```python
from build123d import *

# Parameters (mm, degrees)
SKETCH1_W           = 60
SKETCH1_H           = 400
BOSS_EXTRUDE1_DEPTH = 3
SKETCH2_W           = 3
SKETCH2_H           = 40
SKETCH2_W_2         = 10
SKETCH2_H_2         = 3
SKETCH2_W_3         = 7
SKETCH2_W_4         = 20
CUT_EXTRUDE3_DEPTH  = 3
SKETCH3_W           = 3
SKETCH3_H           = 3
CUT_EXTRUDE4_DEPTH  = 3
SKETCH4_W           = 34
SKETCH4_H           = 20
CUT_EXTRUDE5_DEPTH  = 3
FILLET1_R           = 2


with BuildPart() as part:
    # Sketch1 → Boss-Extrude1 (new body)
    with BuildSketch(Plane.XY):
        Rectangle(SKETCH1_W, SKETCH1_H)
    extrude(amount=BOSS_EXTRUDE1_DEPTH)

    # Sketch2 → Cut-Extrude3 (cut)
    with BuildSketch(Plane.XY.offset(3)):
        with Locations((-28.5, 60)):
            Rectangle(SKETCH2_W, SKETCH2_H)
        with Locations((-28.5, -60)):
            Rectangle(SKETCH2_W, SKETCH2_H)
        with Locations((-28.5, 140)):
            Rectangle(SKETCH2_W, SKETCH2_H)
        with Locations((-28.5, -140)):
            Rectangle(SKETCH2_W, SKETCH2_H)
        with Locations((-15, 198.5)):
            Rectangle(SKETCH2_W_2, SKETCH2_H_2)
        with Locations((-23.5, -198.5)):
            Rectangle(SKETCH2_W_3, SKETCH2_H_2)
        with Locations((15, 198.5)):
            Rectangle(SKETCH2_W_2, SKETCH2_H_2)
        with Locations((0, -198.5)):
            Rectangle(SKETCH2_W_4, SKETCH2_H_2)
        with Locations((23.5, -198.5)):
            Rectangle(SKETCH2_W_3, SKETCH2_H_2)
        with Locations((28.5, 140)):
            Rectangle(SKETCH2_W, SKETCH2_H)
        with Locations((28.5, -140)):
            Rectangle(SKETCH2_W, SKETCH2_H)
        with Locations((28.5, 60)):
            Rectangle(SKETCH2_W, SKETCH2_H)
        with Locations((28.5, -60)):
            Rectangle(SKETCH2_W, SKETCH2_H)
    extrude(amount=-CUT_EXTRUDE3_DEPTH, mode=Mode.SUBTRACT)

    # Sketch3 → Cut-Extrude4 (cut)
    with BuildSketch(Plane.XY.offset(3)):
        with Locations((-28.5, -198.5)):
            Rectangle(SKETCH3_W, SKETCH3_H)
        with Locations((28.5, -198.5)):
            Rectangle(SKETCH3_W, SKETCH3_H)
    extrude(amount=-CUT_EXTRUDE4_DEPTH, mode=Mode.SUBTRACT)

    # Sketch4 → Cut-Extrude5 (cut)
    with BuildSketch(Plane.XY.offset(3)):
        with Locations((0, -167)):
            Rectangle(SKETCH4_W, SKETCH4_H)
        with Locations((0, -127)):
            Rectangle(SKETCH4_W, SKETCH4_H)
        with Locations((0, -87)):
            Rectangle(SKETCH4_W, SKETCH4_H)
        with Locations((0, -47)):
            Rectangle(SKETCH4_W, SKETCH4_H)
        with Locations((0, -7)):
            Rectangle(SKETCH4_W, SKETCH4_H)
        with Locations((0, 33)):
            Rectangle(SKETCH4_W, SKETCH4_H)
        with Locations((0, 73)):
            Rectangle(SKETCH4_W, SKETCH4_H)
        with Locations((0, 113)):
            Rectangle(SKETCH4_W, SKETCH4_H)
    extrude(amount=-CUT_EXTRUDE5_DEPTH, mode=Mode.SUBTRACT)

    # Fillet1
    fillet1_edges = [part.edges().sort_by_distance(p)[0] for p in [
        (17, -157, 1.5),
        (17, -177, 1.5),
        (-17, -177, 1.5),
        (-17, -157, 1.5),
        (17, -117, 1.5),
        (17, -137, 1.5),
        (-17, -137, 1.5),
        (-17, -117, 1.5),
        (17, -77, 1.5),
        (17, -97, 1.5),
        (-17, -97, 1.5),
        (-17, -77, 1.5),
        (17, -37, 1.5),
        (17, -57, 1.5),
        (-17, -57, 1.5),
        (-17, -37, 1.5),
        (17, 3, 1.5),
        (17, -17, 1.5),
        (-17, -17, 1.5),
        (-17, 3, 1.5),
        (17, 43, 1.5),
        (17, 23, 1.5),
        (-17, 23, 1.5),
        (-17, 43, 1.5),
        (17, 83, 1.5),
        (17, 63, 1.5),
        (-17, 63, 1.5),
        (-17, 83, 1.5),
        (17, 123, 1.5),
        (17, 103, 1.5),
        (-17, 103, 1.5),
        (-17, 123, 1.5),
    ]]
    fillet(fillet1_edges, radius=FILLET1_R)


solid = part.part
```
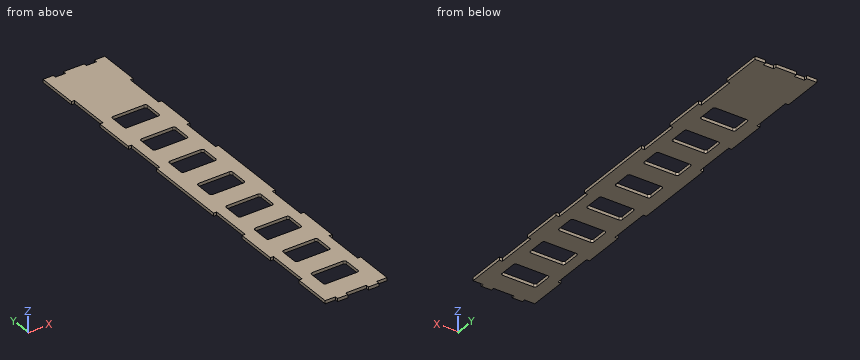
The model under review builds one solid part; all positions refer to its coordinate system, in mm. Round coordinates to 2 decimals unless told otherwise and drop trailing zeros. Loops run counter-clockwise (first coordinate to the right, second up) from the corner with the lowest first, then second, coordinate; pieces in that order, holes last. Notation, with made-up numbers: (-6.75, -31.75) - (0.25, -31.75) arc R35 cw to (0.25, 7.25) - close; hole circle Ø6 at (73.5, 85). An arc over 180 degrees is marked (long way). Use a Markdown table: item, result. Add a question column.
Q1. Add section B-B (y = -49). State the section outline as (x, z) points.
Q2. Insertion check: pin 1 Ø0.9 at (y, z) = (-145, 1) entering from -X; pin 2 Ø0.9 at (y, z) = (-148.5, 2) entering from +X; pin 3 Ø1.5 at (x, z) = (25.5, 1) entering from -Y. Each pin has a flat end and moves straight along its axis. Give the tip position at first contact, or say it passes through.
Q3. Add section A-A (y = 110). State the section outline as (x, z) points.
Q4. Add section C-C (x = -0.5). State how many separate pieces and enclosed holes the cut face has, plus the area to 3 significant figures.
Q5. For probe 1 along X at (y, z) = (74, 0.8); probe 2 along X at (y, z) = (-119.5, 0.6); probe 3 along Y at (x, z) = (-18, 0.1), list the stretches that pass through material, from the lowest coordinate up.
Worked answers:
| question | item | result |
|---|---|---|
| 1 | outline | (-27, 0) - (-17, 0) - (-17, 3) - (-27, 3) - close; (17, 0) - (27, 0) - (27, 3) - (17, 3) - close |
| 2 | pin 1 | x = -27 |
| 2 | pin 2 | x = 27 |
| 2 | pin 3 | y = -197 |
| 3 | outline | (-30, 0) - (-17, 0) - (-17, 3) - (-30, 3) - close; (17, 0) - (30, 0) - (30, 3) - (17, 3) - close |
| 4 | separate pieces | 9 |
| 4 | enclosed holes | 0 |
| 4 | area | 711 mm² |
| 5 | probe 1 | -27 to -17, 17 to 27 |
| 5 | probe 2 | -30 to -17, 17 to 30 |
| 5 | probe 3 | -200 to 197 |
